Check sheet for the drawn part. Datum: minimum x, y, z corner. Units: mm. A direction names the side the tool comes from. Round coordinates to 2 decimals unless told otherwise and drop trailing zeros. Write each loop counter-clockwise with the first axis right and the second up, starting at its lowest first coordinate (ties: lowest second). Pieces come first, ordered by that corner, then holes. Notation, with made-up numbers: (27, 29.25) -> (47, 29.25) arc R24 cw to (47, 45.25) -> close; hole circle Ø4 at (39, 64.25). An arc over 180 degrees is marked (long way). One line per item, written item: value.
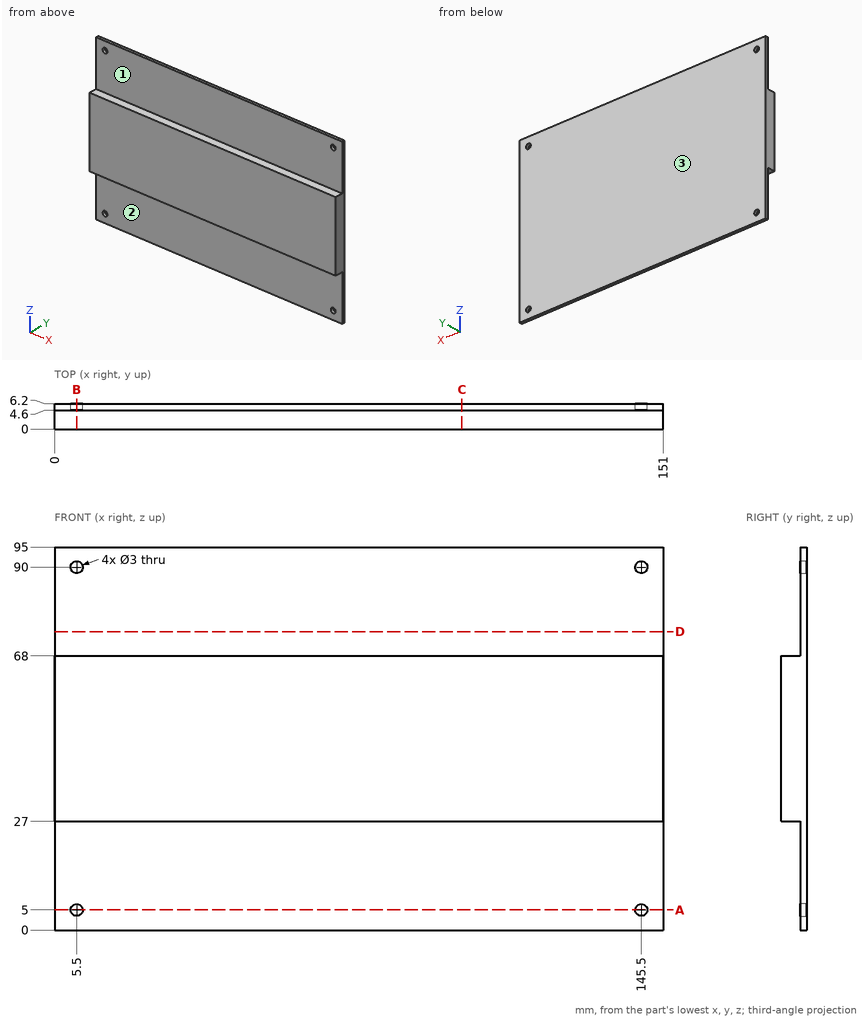
Item 1: Sectioned sample at B-B on x = 5.5. Enter the section's corners in (y, z).
Answer:
outline: (0, 27) -> (4.6, 27) -> (4.6, 6.5) -> (6.2, 6.5) -> (6.2, 88.5) -> (4.6, 88.5) -> (4.6, 68) -> (0, 68) -> close; (4.6, 0) -> (6.2, 0) -> (6.2, 3.5) -> (4.6, 3.5) -> close; (4.6, 91.5) -> (6.2, 91.5) -> (6.2, 95) -> (4.6, 95) -> close
Item 2: Sectioned sample at D-D on z = 74. Enter the section's corners in (x, y), and give its area (3 significant figures).
Answer:
outline: (0, 4.6) -> (151, 4.6) -> (151, 6.2) -> (0, 6.2) -> close
area: 242 mm^2
Item 3: Depth check by flat-ended pin: P1, Ø2.5, axis at x = 57, y = 1.5, coming from the -Z side; P2, Ø8, axis at x = 54.5, z = 81, coming from the -Y side; P3, Ø21.5, axis at x = 70.5, z = 19.5, coming from the -Y side; P4, Ø2, axis at x = 75.5, y = 3, coming from the +Z side. Enter the tip coordinate at first touch or a pass-through.
Answer:
P1: stops at z = 27
P2: stops at y = 4.6
P3: stops at y = 0
P4: stops at z = 68
Item 4: Tool access check on the marked faces 1, 2 and 3. Record the directions out of +Z, -Z, +X, -X, +Y, -Y that give a thin tool (end or side, any length) a straight path to the whole face; none if there is none.
Answer:
face 1: +Z, +X, -X, -Y
face 2: -Z, +X, -X, -Y
face 3: +Z, -Z, +X, -X, +Y
Item 5: Thickness scan on line 1 (X direction, y = 5.6, z = 5); line 2 (Z direction, x = 145.5, y = 5.3); line 3 (Y direction, x = 52, z = 87). Record the ranges inside material, lowest first.
Answer:
line 1: x = 0 to 4, 7 to 144, 147 to 151
line 2: z = 0 to 3.5, 6.5 to 88.5, 91.5 to 95
line 3: y = 4.6 to 6.2
Item 6: Sectioned sample at A-A on z = 5. Enter the section's corners in (x, y), and give its area (3 significant figures).
Answer:
outline: (0, 4.6) -> (4, 4.6) -> (4, 6.2) -> (0, 6.2) -> close; (7, 4.6) -> (144, 4.6) -> (144, 6.2) -> (7, 6.2) -> close; (147, 4.6) -> (151, 4.6) -> (151, 6.2) -> (147, 6.2) -> close
area: 232 mm^2
Item 7: Sectioned sample at C-C on x = 101. Enter the section's corners in (y, z), and give its area (3 significant figures).
Answer:
outline: (0, 27) -> (4.6, 27) -> (4.6, 0) -> (6.2, 0) -> (6.2, 95) -> (4.6, 95) -> (4.6, 68) -> (0, 68) -> close
area: 341 mm^2
